Answer from the drawing. Dimensions are ordinates in mm from the lowest x, y and z of the part. A direction names the side the tool comes from. Give positions to 0.01 mm unless a question says otherwise; leave off trailing zeros. Write each loop counter-clockwise with the first axis right and the second up, starting at its lowest first coordinate (ties: lowest second). Pieces come first, ordered by that corner, then holes. Notation, with made-up numbers: M 42.5,-5.75 L 65.5,-5.75 A18 cw 65.5,14.25 Z; hole C 60.5,-37.75 d10. An arc over 180 degrees is marked long. Put each result on its own line as item: value.
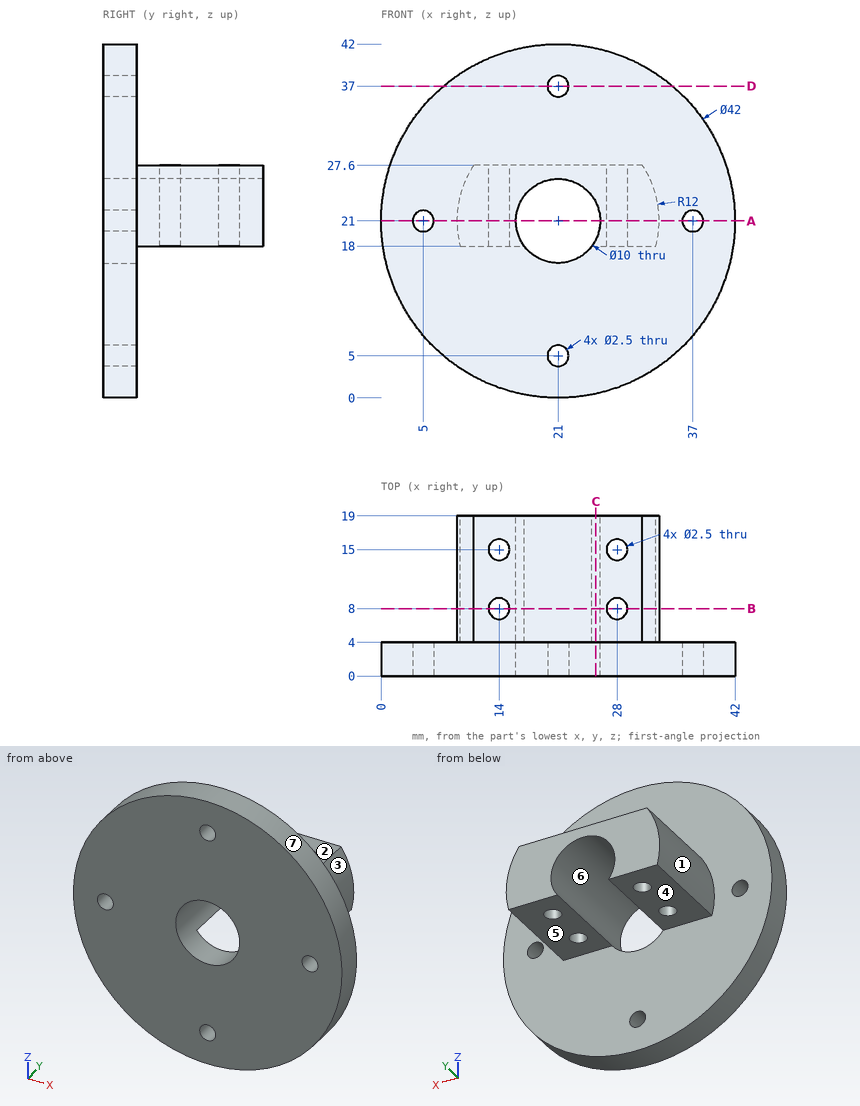
(1) Given pin 1 Ø4 at (x, y) = (12.5, 9) entering from -Z; pin 2 Ø6 at (x, y) = (8, 3) entering from +Z; pin 3 Ø8 at (y, z) = (7.5, 37) entering from -X, each flat-ended and moving along its own axis, determine where each tip first touches the part or whether it passes through.
Result:
pin 1: stops at z = 18
pin 2: stops at z = 39.47
pin 3: stops at x = 5.4
(2) Section D-D on z = 37 is taken. Determine the outline of the cut face in (x, y), and give its area (3 significant figures).
Result:
outline: M 7.4,0 L 19.75,0 L 19.75,4 L 7.4,4 Z; M 22.25,0 L 34.6,0 L 34.6,4 L 22.25,4 Z
area: 98.8 mm²
(3) Straight lines are drawn through the part: line 1 along Y through (x, z) = (14, 24.25); line 2 along X through (y, z) = (12.25, 21); line 3 along X through (y, z) = (8.25, 19.5). For each, find the intervals that lie inside material, in ascending order. Write a range as from..to.
Result:
line 1: y = 0..6.75, 9.25..13.75, 16.25..19
line 2: x = 9..16, 26..33
line 3: x = 9.09..12.78, 15.22..16.23, 25.77..26.78, 29.22..32.91
(4) For a pull along X with two mould halves and no side action, classify the marked faces 5, 6 and 7 as +X half, -X half, draft (parallel to the pull), parting line (faces both ways), or undercut.
Result:
face 5: draft
face 6: undercut
face 7: parting line
(5) Which of the six approach directions +Z, -Z, +X, -X, +Y, -Y give full straight-line access (tool end or side, diameter ignored) to the marked faces 1, 2, 3 and 4?
Result:
face 1: -X, +Y
face 2: +Z, +X, -X, +Y
face 3: +X, +Y
face 4: -Z, +X, -X, +Y
(6) Section A-A on z = 21 is taken. Determine the outline of the cut face in (x, y).
Result:
outline: M 0,0 L 3.75,0 L 3.75,4 L 0,4 Z; M 6.25,0 L 16,0 L 16,19 L 9,19 L 9,4 L 6.25,4 Z; M 26,0 L 35.75,0 L 35.75,4 L 33,4 L 33,19 L 26,19 Z; M 38.25,0 L 42,0 L 42,4 L 38.25,4 Z; hole C 14,8 d2.5; hole C 14,15 d2.5; hole C 28,8 d2.5; hole C 28,15 d2.5
(7) Section B-B on y = 8 is taken. Determine the outline of the cut face in (x, z).
Result:
outline: M 9.38,18 L 12.75,18 L 12.75,27.6 L 10.98,27.6 A12 ccw Z; M 15.25,18 L 17,18 A5 cw long 25,18 L 26.75,18 L 26.75,27.6 L 15.25,27.6 Z; M 29.25,18 L 32.62,18 A12 ccw 31.02,27.6 L 29.25,27.6 Z
(8) Section C-C on x = 25.5 is taken. Determine the outline of the cut face in (y, z).
Result:
outline: M 0,0.49 L 4,0.49 L 4,18 L 19,18 L 19,18.82 L 0,18.82 Z; M 0,23.18 L 19,23.18 L 19,27.6 L 4,27.6 L 4,41.51 L 0,41.51 Z
